Read the model definition and answer for the solid it produces. Units are mm, in the model's axes. Face numbers are marked on the shaded views. Coordinates: 2 decimals unless noted, no trailing zeros. Write each loop counter-clockwise with the first axis right and the second up, starting at its lowest first coordinate (ties: lowest second). Pieces come first, ordered by that corner, then holes.
Item 1: Each of these flat-tipped pins is pushed along its axis until it touches: P1, Ø0.5, axis at y = 848.5, z = -130.5, coming from the -X side; P2, Ø10, axis at y = -42, z = -102.5, coming from the +X side; P3, Ø1, axis at y = -281, z = 190, coming from the +X side. Where does it stop, or does it pass through?
Item 2: Determine the mould class of the marked faces 1, 2, 3 and 4 for opening direction Z: released by +Z, released by -Z, zero draft, split by the parting line, or undercut.
Item 3: Straight lines are drawn through the part: probe 1 along Z at (x, y) = (-73.75, -250); probe 2 along Y at (x, z) = (-74.2, 315.2); probe 3 along Z at (x, y) = (-59.5, 706.5). For each, find the intervals that lie inside material, in ascending order.
Item 4: Section B-B (z = 183) is taken. Give the vertices of the cut face in (x, y).
Item 5: Section C-C (y = 463) is taken. Give the vertices of the cut face in (x, z).
Item 6: Section D-D (x = 22) is taken. Give the vertices of the cut face in (y, z).
Item 7: Section A-A (x = -53) is taken. Give the vertices of the cut face in (y, z).
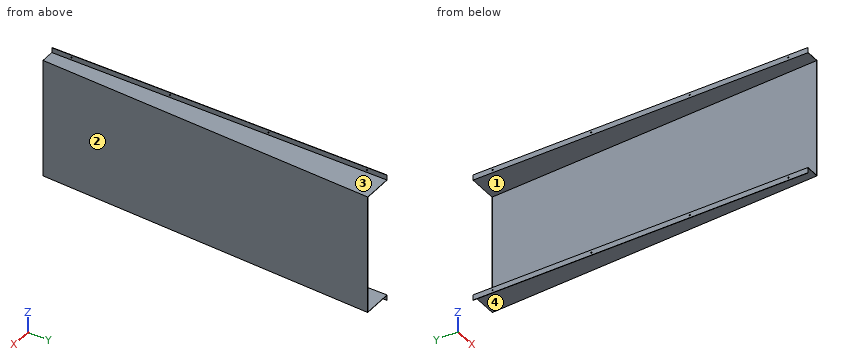
from build123d import *

# Parameters (mm, degrees)
BOSS_EXTRUDE1_DEPTH = 302.5
SHELL1_T            = -1.8
CUT_EXTRUDE4_REACH  = 1730.332
SKETCH22_W          = 148.11330214
SKETCH22_H          = 601.4
CUT_EXTRUDE5_REACH  = 1728.561
SKETCH23_W          = 68.282713905
SKETCH23_H          = 601.4
SKETCH24_W          = 25.4
SKETCH24_H          = 1700
BOSS_EXTRUDE2_DEPTH = 1.8
SKETCH25_R          = 3
CUT_EXTRUDE6_DEPTH  = 10


with BuildPart() as part:
    # Sketch21 → Boss-Extrude1 (new, symmetric)
    with BuildSketch(Plane.XY):
        Polygon((-75, -850), (-75, 850), (75, 850), (-5, -850), align=None)
    extrude(amount=BOSS_EXTRUDE1_DEPTH, both=True)

    # Shell1
    shell1_openings = [part.faces().sort_by_distance(p)[0] for p in [
        (-75, 0, 0),
    ]]
    offset(amount=SHELL1_T, openings=shell1_openings, kind=Kind.INTERSECTION)

    # Sketch22 → Cut-Extrude4 (cut, up to next)
    with BuildSketch(Plane(origin=(0, 850, 0), x_dir=(1, 0, 0), z_dir=(0, 1, 0)), mode=Mode.PRIVATE) as cut_extrude4_sk1:
        with Locations((-0.94334893, 0)):
            Rectangle(SKETCH22_W, SKETCH22_H)
    cut_extrude4_tool1 = extrude(cut_extrude4_sk1.sketch, amount=-CUT_EXTRUDE4_REACH, mode=Mode.PRIVATE) & part.part
    add(cut_extrude4_tool1.solids().sort_by_distance((-0.943349, 850, 0))[0], mode=Mode.SUBTRACT)

    # Sketch23 → Cut-Extrude5 (cut, up to next)
    with BuildSketch(Plane(origin=(0, -848.2, 0), x_dir=(1, 0, 0), z_dir=(0, 1, 0)), mode=Mode.PRIVATE) as cut_extrude5_sk1:
        with Locations((-40.858643048, 0)):
            Rectangle(SKETCH23_W, SKETCH23_H)
    cut_extrude5_tool1 = extrude(cut_extrude5_sk1.sketch, amount=-CUT_EXTRUDE5_REACH, mode=Mode.PRIVATE) & part.part
    add(cut_extrude5_tool1.solids().sort_by_distance((-40.858643, -848.2, 0))[0], mode=Mode.SUBTRACT)

    # Sketch24 → Boss-Extrude2 (add)
    with BuildSketch(Plane.ZY.offset(75)):
        with Locations((-315.2, 0)):
            Rectangle(SKETCH24_W, SKETCH24_H)
        with Locations((315.2, 0)):
            Rectangle(SKETCH24_W, SKETCH24_H)
    extrude(amount=-BOSS_EXTRUDE2_DEPTH)

    # Sketch25 → Cut-Extrude6 (cut)
    with BuildSketch(Plane(origin=(-73.2, 0, 0), x_dir=(0, 0, -1), z_dir=(1, 0, 0))):
        with Locations(Location((-315.2, 750, 0), (0, 0, 90))):
            Circle(SKETCH25_R)
        with Locations(Location((-315.2, 250, 0), (0, 0, 90))):
            Circle(SKETCH25_R)
        with Locations(Location((-315.2, -250, 0), (0, 0, 90))):
            Circle(SKETCH25_R)
        with Locations(Location((-315.2, -750, 0), (0, 0, 90))):
            Circle(SKETCH25_R)
    cut_extrude6 = extrude(amount=-CUT_EXTRUDE6_DEPTH, mode=Mode.SUBTRACT)

    # Mirror1: Cut-Extrude6 across plane
    add(cut_extrude6.mirror(Plane.XY), mode=Mode.SUBTRACT)


solid = part.part
Established:
1. P1: stops at x = 73.11
1. P2: stops at x = 33.26
1. P3: stops at x = 21.8
2. face 1: undercut
2. face 2: zero draft
2. face 3: released by +Z
2. face 4: released by -Z
3. probe 1: z = -327.9 to -318.2, -312.2 to -300.7, 300.7 to 312.2, 318.2 to 327.9
3. probe 2: y = -850 to -753, -747 to -253, -247 to 247, 253 to 747, 753 to 850
3. probe 3: z = -302.5 to -300.7, 300.7 to 302.5
4. outline: (-6.72, -850) - (-5, -850) - (75, 850) - (73.11, 850) - (73.11, 848.2) - (-6.72, -848.2) - close
5. outline: (-75, -327.9) - (-73.2, -327.9) - (-73.2, -302.5) - (56.79, -302.5) - (56.79, 302.5) - (-73.2, 302.5) - (-73.2, 327.9) - (-75, 327.9) - (-75, 300.7) - (54.99, 300.7) - (54.99, -300.7) - (-75, -300.7) - close
6. outline: (-276.25, -302.5) - (850, -302.5) - (850, -300.7) - (-237.96, -300.7) - (-237.96, 300.7) - (850, 300.7) - (850, 302.5) - (-276.25, 302.5) - close
7. outline: (-850, -302.5) - (850, -302.5) - (850, -300.7) - (-850, -300.7) - close; (-850, 300.7) - (850, 300.7) - (850, 302.5) - (-850, 302.5) - close
